Read the model definition and answer for the solid it produces. Units are mm, in the model's axes. Coordinates: 2 decimals unless noted, no trailing zeros. Order: outer loops, then holes, each group sorted by start corner. A loop starts at its lowest first (then second) coordinate and runs counter-clockwise, first axis right, second up. Notation, with made-up numbers: M 31.25,89.25 L 66.25,89.25 A22 ccw 66.25,101.25 Z; hole C 24,-28.75 d3. An arc over 180 degrees is marked long. Use a Markdown table: item, result. Add a question column.
1) Find the intervals of material crossed by probe 1 along Y at (x, z) = (-11, 1.2); probe 2 along Y at (x, z) = (-44.5, 2.3); probe 3 along X at (y, z) = (-18.5, 0.95), in increasing order. Write a range as [from, to].
2) Find section C-C on x = -99.5. Write down the section's boundary in (y, z).
3) Find section A-A on x = -34.5. Write down the section's boundary in (y, z).
4) Find section D-D on z = 1.1. Count the separate pieces of the cut face and the enclosed holes in it, plus the area to 3 significant figures.
5) Each of these flat-tipped pins is pushed along its axis until it touches: pin 1 Ø0.9 at (y, z) = (-24, 2) entering from -X; pin 2 Ø1.5 at (x, z) = (-123.5, 1.5) entering from +Y; pin 3 Ø10 at (x, y) = (100.5, -18.5) entering from -Z; pin 4 Ø1.5 at (y, z) = (23, 1.5) entering from +X. Where does it stop, or does it pass through?
6) Find section B-B on y = 10. Write down the section's boundary in (x, z), plus the area to 3 significant figures.
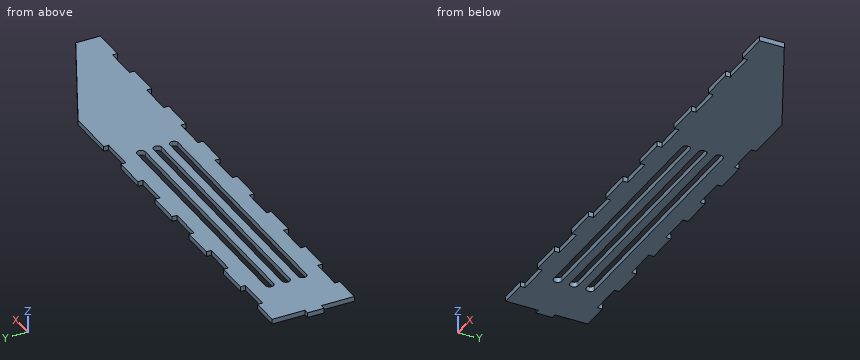
from build123d import *

# Parameters (mm, degrees)
BOSS_EXTRUDE1_DEPTH = 3
SKETCH2_W           = 20
SKETCH2_H           = 3
SKETCH2_W_2         = 3
SKETCH2_H_2         = 10
CUT_EXTRUDE1_DEPTH  = 3
SKETCH3_W           = 3
SKETCH3_H           = 10
CUT_EXTRUDE2_DEPTH  = 3
CUT_EXTRUDE3_DEPTH  = 3


with BuildPart() as part:
    # Sketch1 → Boss-Extrude1 (new body)
    with BuildSketch(Plane.XY):
        Polygon((80, 25), (150, -10), (150, -25), (-150, -25), (-150, 25), align=None)
    extrude(amount=BOSS_EXTRUDE1_DEPTH)

    # Sketch2 → Cut-Extrude1 (cut)
    with BuildSketch(Plane.XY.offset(3)):
        with Locations((-120, 23.5)):
            Rectangle(SKETCH2_W, SKETCH2_H)
        with Locations((-80, 23.5)):
            Rectangle(SKETCH2_W, SKETCH2_H)
        with Locations((-40, 23.5)):
            Rectangle(SKETCH2_W, SKETCH2_H)
        with Locations((-148.5, 10)):
            Rectangle(SKETCH2_W_2, SKETCH2_H_2)
        with Locations((-120, -23.5)):
            Rectangle(SKETCH2_W, SKETCH2_H)
        with Locations((0, 23.5)):
            Rectangle(SKETCH2_W, SKETCH2_H)
        with Locations((40, 23.5)):
            Rectangle(SKETCH2_W, SKETCH2_H)
        with Locations((-80, -23.5)):
            Rectangle(SKETCH2_W, SKETCH2_H)
        with Locations((-40, -23.5)):
            Rectangle(SKETCH2_W, SKETCH2_H)
        with Locations((0, -23.5)):
            Rectangle(SKETCH2_W, SKETCH2_H)
        with Locations((40, -23.5)):
            Rectangle(SKETCH2_W, SKETCH2_H)
        with Locations((80, -23.5)):
            Rectangle(SKETCH2_W, SKETCH2_H)
        with Locations((120, -23.5)):
            Rectangle(SKETCH2_W, SKETCH2_H)
        with Locations((-148.5, -10)):
            Rectangle(SKETCH2_W_2, SKETCH2_H_2)
    extrude(amount=-CUT_EXTRUDE1_DEPTH, mode=Mode.SUBTRACT)

    # Sketch3 → Cut-Extrude2 (cut)
    with BuildSketch(Plane.XY.offset(3)):
        with Locations((-148.5, 20)):
            Rectangle(SKETCH3_W, SKETCH3_H)
        with Locations((-148.5, -20)):
            Rectangle(SKETCH3_W, SKETCH3_H)
    extrude(amount=-CUT_EXTRUDE2_DEPTH, mode=Mode.SUBTRACT)

    # Sketch4 → Cut-Extrude3 (cut)
    with BuildSketch(Plane.XY.offset(3)):
        with BuildLine():
            Line((35, 7.5), (-115, 7.5))
            ThreePointArc((-115, 7.5), (-117.5, 10), (-115, 12.5))
            Line((-115, 12.5), (35, 12.5))
            ThreePointArc((35, 12.5), (37.5, 10), (35, 7.5))
        make_face()
        with BuildLine():
            Line((35, -2.5), (-115, -2.5))
            ThreePointArc((-115, -2.5), (-117.5, 0), (-115, 2.5))
            Line((-115, 2.5), (35, 2.5))
            ThreePointArc((35, 2.5), (37.5, 0), (35, -2.5))
        make_face()
        with BuildLine():
            Line((35, -12.5), (-115, -12.5))
            ThreePointArc((-115, -12.5), (-117.5, -10), (-115, -7.5))
            Line((-115, -7.5), (35, -7.5))
            ThreePointArc((35, -7.5), (37.5, -10), (35, -12.5))
        make_face()
    extrude(amount=-CUT_EXTRUDE3_DEPTH, mode=Mode.SUBTRACT)


solid = part.part
Check result:
| question | item | result |
|---|---|---|
| 1 | probe 1 | y = [-25, -12.5], [-7.5, -2.5], [2.5, 7.5], [12.5, 25] |
| 1 | probe 2 | y = [-22, -12.5], [-7.5, -2.5], [2.5, 7.5], [12.5, 22] |
| 1 | probe 3 | x = [-147, 150] |
| 2 | outline | M -25,0 L -12.5,0 L -12.5,3 L -25,3 Z; M -7.5,0 L -2.5,0 L -2.5,3 L -7.5,3 Z; M 2.5,0 L 7.5,0 L 7.5,3 L 2.5,3 Z; M 12.5,0 L 25,0 L 25,3 L 12.5,3 Z |
| 3 | outline | M -22,0 L -12.5,0 L -12.5,3 L -22,3 Z; M -7.5,0 L -2.5,0 L -2.5,3 L -7.5,3 Z; M 2.5,0 L 7.5,0 L 7.5,3 L 2.5,3 Z; M 12.5,0 L 22,0 L 22,3 L 12.5,3 Z |
| 4 | separate pieces | 1 |
| 4 | enclosed holes | 3 |
| 4 | area | 10,600 mm2 |
| 5 | pin 1 | stops at x = -147 |
| 5 | pin 2 | stops at y = 22 |
| 5 | pin 3 | stops at z = 0 |
| 5 | pin 4 | stops at x = 85.5 |
| 6 | outline | M -147,0 L -117.5,0 L -117.5,3 L -147,3 Z; M 37.5,0 L 110,0 L 110,3 L 37.5,3 Z |
| 6 | area | 306 mm2 |
